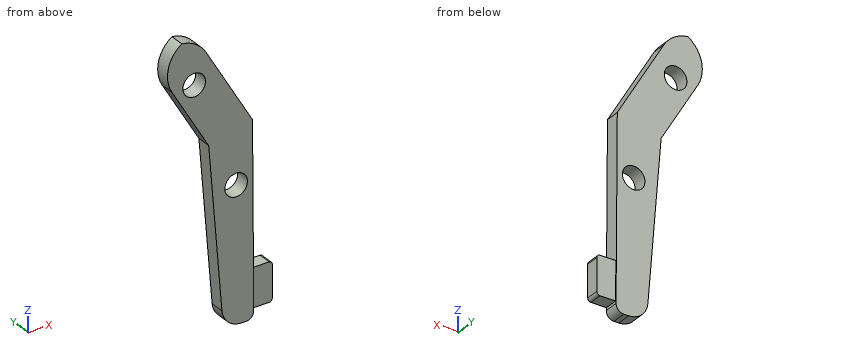
```python
from build123d import *

# Parameters (mm, degrees)
BOSS_EXTRUDE1_DEPTH = 2.25
FILLET1_R           = 5
BOSS_EXTRUDE2_REACH = 40.996
SKETCH4_W           = 6
SKETCH4_H           = 2.1
SKETCH4_2_W         = 6
SKETCH4_2_H         = 2.1
BOSS_EXTRUDE3_DEPTH = 2.908330475
FILLET2_R           = 3
FILLET3_R           = 1.2
FILLET4_R           = 0.5
SKETCH2_R           = 1.75
CUT_EXTRUDE1_DEPTH  = 10


with BuildPart() as part:
    # Sketch1 → Boss-Extrude1 (new body)
    with BuildSketch(Plane(origin=(0, 0, 0), x_dir=(1, 0, 0), z_dir=(0, 1, 0))):
        Polygon((0, 0), (9.103642727, 15.528157943), (11.383305122, 43.435202562), (16.102594303, 43.435202562), (15.904357834, 13.869762926), (6.800715107, -1.658395017), align=None)
    extrude(amount=BOSS_EXTRUDE1_DEPTH)

    # Fillet1
    # the kernel refuses this fillet: 5 mm, written as the material it takes off along each edge
    with BuildSketch(Plane(origin=(6.800715107, -9.304114403, 1.658395017), x_dir=(0.5057579292685198, 0, -0.8626754412767405), z_dir=(0, 1, 0))) as fillet1_piece_1:
        with BuildLine():
            CenterArc((FILLET1_R * 0.744329152265, FILLET1_R), FILLET1_R, 196.677230039, 73.322769961)
            Line((-FILLET1_R * 0.213607467111, FILLET1_R * 0.713020151823), (0, 0))
            Line((0, 0), (FILLET1_R * 0.744329152265, 0))
        make_face()
    extrude(amount=20.858228807, mode=Mode.SUBTRACT)
    with BuildSketch(Plane(origin=(0, -16.79364561, 0), x_dir=(0.5057579292685198, 0, -0.8626754412767405), z_dir=(0, 1, 0))) as fillet1_piece_2:
        with BuildLine():
            CenterArc((FILLET1_R * 1.34349164877, -FILLET1_R), FILLET1_R, 90, 106.677230039)
            Line((FILLET1_R * 0.38555502939, -FILLET1_R * 1.28697984818), (0, 0))
            Line((0, 0), (FILLET1_R * 1.34349164877, 0))
        make_face()
    extrude(amount=35.837291219, mode=Mode.SUBTRACT)

    # Boss-Extrude2: up to this plane
    boss_extrude2_end = Plane(origin=(15.904357834, 2.25, -13.869762926), z_dir=(-0.9999775222008104, 0, -0.006704855936389689))
    # Sketch4 → Boss-Extrude2 (add, up to the surface)
    with BuildSketch(Plane(origin=(19, -1.484709168, -8.201879583), x_dir=(0, 0, -1), z_dir=(1, 0, 0)), mode=Mode.PRIVATE) as boss_extrude2_sk1:
        with Locations((30.603976534, 2.57086864)):
            Rectangle(SKETCH4_W, SKETCH4_H)
    boss_extrude2_tool1 = split(extrude(boss_extrude2_sk1.sketch, amount=-BOSS_EXTRUDE2_REACH, mode=Mode.PRIVATE), bisect_by=boss_extrude2_end, keep=Keep.BOTH, mode=Mode.PRIVATE)
    add(boss_extrude2_tool1.solids().sort_by_distance((19, 1.086159, -38.805856))[0])

    # Sketch4<2> → Boss-Extrude3 (add)
    with BuildSketch(Plane(origin=(19, -1.484709168, -8.201879583), x_dir=(0, 0, -1), z_dir=(1, 0, 0))):
        with Locations((30.603976534, 2.57086864)):
            Rectangle(SKETCH4_2_W, SKETCH4_2_H)
    extrude(amount=-BOSS_EXTRUDE3_DEPTH)

    # Fillet2
    fillet2_edges = [part.edges().sort_by_distance(p)[0] for p in [
        (11.383305122, 1.125, -43.435202562),
    ]]
    fillet(fillet2_edges, radius=FILLET2_R)

    # Fillet3
    fillet3_edges = [part.edges().sort_by_distance(p)[0] for p in [
        (16.102594303, 1.125, -43.435202562),
    ]]
    fillet(fillet3_edges, radius=FILLET3_R)

    # Fillet4
    fillet4_edges = [part.edges().sort_by_distance(p)[0] for p in [
        (19, 1.086159472, -41.805856117),
        (19, 1.086159472, -35.805856117),
    ]]
    fillet(fillet4_edges, radius=FILLET4_R)

    # Sketch2 → Cut-Extrude1 (cut)
    with BuildSketch(Plane(origin=(0, 2.25, 0), x_dir=(1, 0, 0), z_dir=(0, 1, 0))):
        with Locations(Location((6.857494693, 5.853068737, 0), (0, 0, 270))):
            Circle(SKETCH2_R)
        with Locations(Location((13.362356268, 22.747397122, 0), (0, 0, 270))):
            Circle(SKETCH2_R)
    extrude(amount=-CUT_EXTRUDE1_DEPTH, mode=Mode.SUBTRACT)


solid = part.part
```
The model under review builds one solid part; all positions refer to its coordinate system, in mm. Give positions to 0.01 mm unless a question says otherwise; leave off trailing zeros. Write each loop counter-clockwise with the first axis right and the second up, starting at its lowest first coordinate (ties: lowest second). Pieces come first, ordered by that corner, then holes. Notation, with made-up numbers: M 50,-5 L 61,-5 A12 ccw 61,17 Z; hole C 33.25,50 d6. An arc over 180 degrees is marked long. Write item = value, one per line. Start each with the question number.
Q1. For line 1 (X direction, y = 0.3, z = -6.5); line 2 (Z direction, x = 14.25, y = 0.25); line 3 (Z direction, x = 5.75, y = 0.2), list the stretches that pass through material, from the lowest coordinate up.
Q2. We need section A-A (x = 8). State the section outline as (y, z) points, plus the area to 3 significant figures.
Q3. Clearance check with flat-ended pins moving along their axes: pin 1 (3 mm diameter, centred on x = 18, z = -39, fed in from -Y); pin 2 (1 mm diameter, centred on x = 17.5, y = 1, fed in from +Z); pin 3 (2 mm diameter, centred on x = 6.86, z = -5.85, fed in from -Y); pin 4 (1.5 mm diameter, centred on x = 17.5, z = -39, fed in from +Y). State where each tip first meets the part, or that it passes through.
Q4. We need section B-B (z = -23). State the section outline as (x, y) points.
Q5. We need section C-C (y = 1.75). State the section outline as (x, z) points.
Result set:
q1.line_1 = 3.81 to 5.23, 8.48 to 11.58
q1.line_2 = -43.44 to -24.26, -21.24 to -11.05
q1.line_3 = -9.81 to -7.21, -4.5 to 0.72
q2.outline = M 0,-13.65 L 2.25,-13.65 L 2.25,-7.18 L 0,-7.18 Z; M 0,-4.53 L 2.25,-4.53 L 2.25,-0.64 L 0,-0.64 Z
q2.area = 23.3 mm2
q3.pin_1 = 0.04
q3.pin_2 = -35.81
q3.pin_3 = through
q3.pin_4 = 2.14
q4.outline = M 9.71,0 L 11.63,0 L 11.63,2.25 L 9.71,2.25 Z; M 15.09,0 L 15.97,0 L 15.97,2.25 L 15.09,2.25 Z
q5.outline = M 3.4,-5.79 L 9.1,-15.53 L 11.16,-40.68 A3 ccw 14.15,-43.44 L 14.89,-43.44 A1.2 ccw 16.09,-42.23 L 16.09,-41.81 L 18.5,-41.81 A0.5 ccw 19,-41.31 L 19,-36.31 A0.5 ccw 18.5,-35.81 L 16.05,-35.81 L 15.9,-13.87 L 8.68,-1.55 A5 ccw 4.93,0.89 A5 ccw Z; hole C 6.86,-5.85 d3.5; hole C 13.36,-22.75 d3.5
